```python
from build123d import *

# Parameters (mm, degrees)
F1_DEPTH = 30
F2_R     = 1
F3_R     = 2
F5_DEPTH = 30
F6_R     = 1
F8_DEPTH = 30
F9_R     = 2


with BuildPart() as f1:
    # F0 (on Right) → F1 (new body)
    with BuildSketch(Plane.YZ):
        with BuildLine():
            ThreePointArc((-8.9644660941, 39.6406786749), (-12.5, 31.105144769), (-16.0355339059, 39.6406786749))
            Line((-16.0355339059, 39.6406786749), (-18.8639610307, 42.4691057996))
            ThreePointArc((-18.8639610307, 42.4691057996), (-20.4235610781, 40.373303604), (-21.3155532551, 37.9178832515))
            Line((-21.3155532551, 37.9178832515), (-25, 20))
            Line((-25, 20), (0, 20))
            Line((0, 20), (-3.6844467449, 37.9178832515))
            ThreePointArc((-3.6844467449, 37.9178832515), (-4.5764389219, 40.373303604), (-6.1360389693, 42.4691057996))
            Line((-6.1360389693, 42.4691057996), (-8.9644660941, 39.6406786749))
        make_face()
    extrude(amount=F1_DEPTH)

    # F2
    f2_edges = [f1.edges().sort_by_distance(p)[0] for p in [
        (15, -8.964466, 39.640679),
        (15, -16.035534, 39.640679),
    ]]
    fillet(f2_edges, radius=F2_R)

    # F3
    f3_edges = [f1.edges().sort_by_distance(p)[0] for p in [
        (15, -6.136039, 42.469106),
        (15, -18.863961, 42.469106),
    ]]
    fillet(f3_edges, radius=F3_R)

    # F4 (on face) → F5 (cut, through all)
    with BuildSketch(Plane.YZ.offset(30)):
        with BuildLine():
            Line((-19.910434928, 29.8565414207), (-21.3203426366, 23))
            Line((-21.3203426366, 23), (-3.6796573634, 23))
            Line((-3.6796573634, 23), (-5.089565072, 29.8565414207))
            add(Edge.make_bspline(
                [(-19.910434928, 29.8565414207), (-17.6130099069, 27.8782596362), (-12.4507025539, 27.4679496916), (-7.4855849853, 27.8458202643), (-5.089565072, 29.8565414207)],
                knots=[0, 0, 0, 0, 0.5, 1, 1, 1, 1], degree=3))
        make_face()
    extrude(amount=-F5_DEPTH, mode=Mode.SUBTRACT)

    # F6
    f6_edges = [f1.edges().sort_by_distance(p)[0] for p in [
        (15, -21.320343, 23),
        (15, -19.910435, 29.856541),
        (15, -3.679657, 23),
        (15, -5.089565, 29.856541),
    ]]
    fillet(f6_edges, radius=F6_R)

    # F7 (on face) → F8 (cut, through all)
    with BuildSketch(Plane.YZ.offset(30)):
        with BuildLine():
            ThreePointArc((-3.1383199654, 35.2620066566), (-4.2638904774, 33.5537090418), (-2.5555928626, 32.4281385298))
            Line((-2.5555928626, 32.4281385298), (-3.1383199654, 35.2620066566))
        make_face()
        with BuildLine():
            ThreePointArc((-22.4444071374, 32.4281385298), (-21.2389555005, 32.7238956084), (-20.7064631841, 33.8450725932))
            ThreePointArc((-20.7064631841, 33.8450725932), (-21.0318666012, 34.7591606787), (-21.8616800346, 35.2620066566))
            Line((-21.8616800346, 35.2620066566), (-22.4444071374, 32.4281385298))
        make_face()
    extrude(amount=-F8_DEPTH, mode=Mode.SUBTRACT)

    # F9
    f9_edges = [f1.edges().sort_by_distance(p)[0] for p in [
        (15, -21.86168, 35.262007),
        (15, -22.444407, 32.428139),
        (15, -3.13832, 35.262007),
        (15, -2.555593, 32.428139),
    ]]
    fillet(f9_edges, radius=F9_R)


solid = f1.part
```
CAD build for the part. Positions are in the model's coordinates, mm. A direction names the side the tool comes from. Coordinates: 2 decimals unless noted, no trailing zeros. Write each loop counter-clockwise with the first axis right and the second up, starting at its lowest first coordinate (ties: lowest second). Pieces come first, ordered by that corner, then holes.
(1) Drill centre lines: probe 1 along Z at (x, y) = (11.5, -18.75); probe 2 along Y at (x, z) = (27, 34.5); probe 3 along Z at (x, y) = (18, -13.5). Where is each one in solid material? Low to high.
(2) Flat gauge pins, fed straight in: pin 1 (5 mm diameter, centred on x = 19.5, z = 33, fed in from +Y); pin 2 (1 mm diameter, centred on y = -6, z = 23, fed in from -X); pin 3 (6 mm diameter, centred on x = 16, z = 33, fed in from -Y); pin 4 (1 mm diameter, centred on x = 10, z = 34.5, fed in from +Y). Where does each tip first touch, or does it go through?
(3) 3-axis set-ups, long thin cutter, end or side, ignore diameter. For faces 1 (the face through (30, -13, 28)), 2 (the face through (14.79, -20.88, 23.38)): which of +Z, -Z, +X, -X, +Y, -Y reach the whole face in a straight line?
(4) Cut at A-A, the plane z = 26. List the corners of the cut face in (x, y), and give its area (3 significant figures).
(5) Cut at B-B, the plane z = 21.5. List the corners of the cut face in (x, y), and give its area (3 significant figures).
(6) Two-plate mould, pull along Y, no slides. Class faces 3 (the face through (15.21, -18.921, 41.417)), 4 (the face through (14.79, -3.546, 37.247)), 5 (the face through (15.21, -8.607, 39.655)), 6 (the face through (14.79, -21.55, 35.64)): +Y half, -Y half, draft (parallel to the pull), parting line (faces both ways), or undercut.
Geometry says:
1. probe 1: z = 20 to 23, 29.01 to 41.43
1. probe 2: y = -20.86 to -17.24, -7.76 to -4.14
1. probe 3: z = 20 to 23, 27.68 to 31.21
2. pin 1: stops at y = -2.16
2. pin 2: stops at x = 0
2. pin 3: stops at y = -22.94
2. pin 4: stops at y = -3.77
3. face 1: +Z, -Z, +X, +Y, -Y
3. face 2: +X, -X
4. outline: (0, -23.77) - (30, -23.77) - (30, -20.7) - (0, -20.7) - close; (0, -4.3) - (30, -4.3) - (30, -1.23) - (0, -1.23) - close
4. area: 184 mm2
5. outline: (0, -24.69) - (30, -24.69) - (30, -0.31) - (0, -0.31) - close
5. area: 731 mm2
6. face 3: undercut
6. face 4: +Y half
6. face 5: undercut
6. face 6: -Y half
